For this review, take the finished solid that the model builds, in its own axes (mm). Face numbers are marked on the shaded views. A direction names the side the tool comes from. Round coordinates to 2 decimals unless told otherwise and drop trailing zeros. Order: outer loops, then holes, each group sorted by start corner. A loop starts at its lowest first (then second) coordinate and runs counter-clockwise, first axis right, second up.
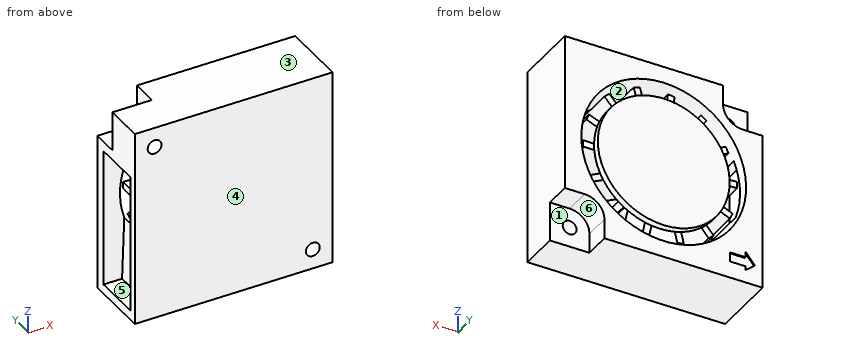
```python
from build123d import *

# Parameters (mm, degrees)
SKETCH_1_W               = 30
SKETCH_1_H               = 30
EXTRUDE_1_DEPTH          = 10
SKETCH_2_W               = 6
SKETCH_2_H               = 6
CUT_EXTRUDE_1_DEPTH      = 4
SKETCH_3_R               = 12.5
CUT_EXTRUDE_2_DEPTH      = 8
FILLET_1_R               = 3
FILLET_2_R               = 3
CUT_EXTRUDE_3_DEPTH      = 0.2
SKETCH_5_R               = 1.05
CUT_EXTRUDE_4_DEPTH      = 10
SKETCH_6_W               = 11.699783002
SKETCH_6_H               = 1
EXTRUDE_2_DEPTH          = 7
PATTERN_CIRCULAR_1_COUNT = 14
PATTERN_CIRCULAR_1_ANGLE = 338
CUT_EXTRUDE_6_REACH      = 45.589
SKETCH_8_W               = 21.07962881
SKETCH_8_H               = 7.180633791
SKETCH_7_R               = 10
EXTRUDE_3_DEPTH          = 1


with BuildPart() as part:
    # 草图1 → 凸台-拉伸1 (new body)
    with BuildSketch(Plane(origin=(0, 0, 0), x_dir=(1, 0, 0), z_dir=(0, 1, 0))):
        with Locations((15, -15)):
            Rectangle(SKETCH_1_W, SKETCH_1_H)
    extrude(amount=EXTRUDE_1_DEPTH)

    # 草图2 → 切除-拉伸1 (cut)
    with BuildSketch(Plane(origin=(0, 10, 0), x_dir=(1, 0, 0), z_dir=(0, 1, 0))):
        with Locations((3, -27)):
            Rectangle(SKETCH_2_W, SKETCH_2_H)
        with Locations((27, -3)):
            Rectangle(SKETCH_2_W, SKETCH_2_H)
    extrude(amount=-CUT_EXTRUDE_1_DEPTH, mode=Mode.SUBTRACT)

    # 草图3 → 切除-拉伸2 (cut)
    with BuildSketch(Plane(origin=(0, 10, 0), x_dir=(1, 0, 0), z_dir=(0, 1, 0))):
        with Locations(Location((15, -15, 0), (0, 0, 270))):
            Circle(SKETCH_3_R)
    extrude(amount=-CUT_EXTRUDE_2_DEPTH, mode=Mode.SUBTRACT)

    # 圆角1
    fillet_1_edges = [part.edges().sort_by_distance(p)[0] for p in [
        (6, 8, 24),
    ]]
    fillet(fillet_1_edges, radius=FILLET_1_R)

    # 圆角2
    fillet_2_edges = [part.edges().sort_by_distance(p)[0] for p in [
        (24, 8, 6),
    ]]
    fillet(fillet_2_edges, radius=FILLET_2_R)

    # 草图4 → 切除-拉伸3 (cut)
    with BuildSketch(Plane(origin=(0, 10, 0), x_dir=(1, 0, 0), z_dir=(0, 1, 0))):
        Polygon((2.568201557, -1.964971172), (1.165606626, -3.118215893), (2.568201557, -4.824074593), (2.568201557, -3.971145243), (4.983781716, -3.971145243), (4.983781716, -2.541593533), (2.568201557, -2.541593533), align=None)
    extrude(amount=-CUT_EXTRUDE_3_DEPTH, mode=Mode.SUBTRACT)

    # 草图5 → 切除-拉伸4 (cut)
    with BuildSketch(Plane(origin=(0, 6, 0), x_dir=(1, 0, 0), z_dir=(0, 1, 0))):
        with Locations(Location((3, -27, 0), (0, 0, 270))):
            Circle(SKETCH_5_R)
        with Locations(Location((27, -3, 0), (0, 0, 270))):
            Circle(SKETCH_5_R)
    extrude(amount=-CUT_EXTRUDE_4_DEPTH, mode=Mode.SUBTRACT)

    # 草图6 → 凸台-拉伸2 (add)
    with BuildSketch(Plane(origin=(0, 2, 0), x_dir=(1, 0, 0), z_dir=(0, 1, 0))):
        with Locations((20.849891501, -14.693219625)):
            Rectangle(SKETCH_6_W, SKETCH_6_H)
    extrude_2 = extrude(amount=EXTRUDE_2_DEPTH)

    # 阵列(圆周)1: 凸台-拉伸2 ×14 about axis
    pattern_circular_1_axis = Axis((15, 0, 15), (0, 1, 0))
    for i in range(1, PATTERN_CIRCULAR_1_COUNT):
        add(extrude_2.rotate(pattern_circular_1_axis, i * PATTERN_CIRCULAR_1_ANGLE / (PATTERN_CIRCULAR_1_COUNT - 1)))

    # 切除-拉伸6: up to this plane
    cut_extrude_6_end = Plane(origin=(3.335500419, 9, 16.214605444), z_dir=(0.9993908270190957, 0, -0.034899496702506666))
    # 草图8 → 切除-拉伸6 (cut, up to the surface)
    with BuildSketch(Plane.ZY, mode=Mode.PRIVATE) as cut_extrude_6_sk1:
        with Locations((11.979819264, 4.784272805)):
            Rectangle(SKETCH_8_W, SKETCH_8_H)
    cut_extrude_6_tool1 = split(extrude(cut_extrude_6_sk1.sketch, amount=-CUT_EXTRUDE_6_REACH, mode=Mode.PRIVATE), bisect_by=cut_extrude_6_end, keep=Keep.BOTH, mode=Mode.PRIVATE)
    add(cut_extrude_6_tool1.solids().sort_by_distance((0, 4.784273, 11.979819))[0], mode=Mode.SUBTRACT)

    # 草图7 → 凸台-拉伸3 (add)
    with BuildSketch(Plane(origin=(0, 9, 0), x_dir=(1, 0, 0), z_dir=(0, 1, 0))):
        with Locations(Location((15, -15, 0), (0, 0, 82.627540404))):
            Circle(SKETCH_7_R)
    extrude(amount=EXTRUDE_3_DEPTH)


solid = part.part
```
Q1. Tool access review of the marked faces 4, 5 and 6: name each direction out of +Z, -Z, +X, -X, +Y, -Y from which nothing blocks a thin tool from reaching the whole face with its end or side.
Q2. Take a section at A-A, the plane x = 20. Count the separate pieces of the cut face and the enclosed holes in it, plus the area to 3 significant figures.
Q3. Mouldability with a two-part tool opening along Z and no side actions: class the marked faces 1, 2 and 3 as +Z half, -Z half, draft (parallel to the pull), parting line (faces both ways), or undercut.
Q4. Take a section at C-C, the plane x = 15. State the section outline as (y, z) points, plus the area to 3 significant figures.
Q5. Take a section at B-B, the plane z = 25.5. State the section outline as (x, y) points.
Q6. Clearance check with flat-ended pins moving along their axes: pin 1 (0.7 mm diameter, centred on x = 18, z = 25.5, fed in from +Y); pin 2 (1 mm diameter, centred on y = 6, z = 17.5, fed in from -X); pin 3 (3 mm diameter, centred on x = 2, z = 28, fed in from +Y). State where each tip first meets the part, or that it passes through.
Q7. Wall thickness on line 1 (Y direction, x = 17, z = 18.5); line 2 (X direction, y = 7.5, z = 7.5); line 3 (X direction, y = 6.25, z = 8.25): over which ranges is each line inside the solid? List them lowest first.
Working result:
1. face 4: +Z, -Z, +X, -X, -Y
1. face 5: -X
1. face 6: -Z, +X, +Y
2. separate pieces: 1
2. enclosed holes: 4
2. area: 178 mm2
3. face 1: draft
3. face 2: undercut
3. face 3: +Z half
4. outline: (0, 0) - (10, 0) - (10, 2.5) - (2, 2.5) - (2, 11.12) - (9, 11.12) - (9, 5) - (10, 5) - (10, 25) - (9, 25) - (9, 19.65) - (2, 19.65) - (2, 27.5) - (10, 27.5) - (10, 30) - (0, 30) - close
4. area: 180 mm2
5. outline: (0, 0) - (30, 0) - (30, 10) - (21.78, 10) - (21.78, 2) - (18.85, 2) - (18.85, 9) - (17.81, 9) - (17.81, 2) - (13.97, 2) - (13.97, 9) - (12.95, 9) - (12.95, 2) - (8.22, 2) - (8.22, 10) - (5.6, 10) - (5.6, 6) - (0, 6) - close
6. pin 1: stops at y = 9
6. pin 2: stops at x = 8.95
6. pin 3: stops at y = 6
7. line 1: y = 0 to 2, 9 to 10
7. line 2: x = 3.03 to 5, 7.65 to 8.96, 12.3 to 13.33, 15.77 to 16.79, 19.84 to 21.1, 25 to 30
7. line 3: x = 3.06 to 4.48, 8.28 to 9.59, 12.49 to 13.52, 15.61 to 16.63, 19.25 to 20.52, 25.52 to 30
